```python
from build123d import *

# Parameters (mm, degrees)
CHANFREIN1_SIZE         = 3
CHANFREIN1_SIZE2        = 1.091910703
CONG_1_R                = 2
ENL_V_MAT_EXTRU_1_DEPTH = 3
ESQUISSE3_R             = 1.5
ENL_V_MAT_EXTRU_2_DEPTH = 3
ESQUISSE4_R             = 5
ESQUISSE4_R_2           = 1.5
ENL_V_MAT_EXTRU_3_DEPTH = 1


with BuildPart() as part:
    # Esquisse1 → Révolution1 (revolve)
    with BuildSketch(Plane.XY):
        Polygon((0, 23), (0, -20), (0, -22), (-1.5, -22), (-1.5, -20), (-15, -20), (-15, 5), (-5, 5), (-5, 10), (-1.5, 10), (-1.5, 23), align=None)
    revolve(axis=Axis((0, 23, 0), (0, -1, 0)))

    # Chanfrein1
    chanfrein1_edges = [part.edges().sort_by_distance(p)[0] for p in [
        (15, 5, 0),
    ]]
    chanfrein1_side = [part.faces().sort_by_distance(p)[0] for p in [
        (15, -7.5, 0),
    ]]
    chamfer(chanfrein1_edges, length=CHANFREIN1_SIZE, length2=CHANFREIN1_SIZE2, reference=chanfrein1_side[0])

    # Congé1
    cong_1_edges = [part.edges().sort_by_distance(p)[0] for p in [
        (15, -20, 0),
    ]]
    fillet(cong_1_edges, radius=CONG_1_R)

    # Esquisse2 → Enlèv. mat.-Extru.1 (cut)
    with BuildSketch(Plane(origin=(0, 5, 0), x_dir=(1, 0, 0), z_dir=(0, 1, 0))):
        with BuildLine():
            Line((-4, 9), (-4, 19))
            Line((-4, 19), (4, 19))
            Line((4, 19), (4, 9))
            ThreePointArc((4, 9), (0, 5), (-4, 9))
        make_face()
        with BuildLine():
            Line((9, 4), (19, 4))
            Line((19, 4), (19, -4))
            Line((19, -4), (9, -4))
            ThreePointArc((9, -4), (5, 0), (9, 4))
        make_face()
        with BuildLine():
            Line((4, -9), (4, -19))
            Line((4, -19), (-4, -19))
            Line((-4, -19), (-4, -9))
            ThreePointArc((-4, -9), (0, -5), (4, -9))
        make_face()
        with BuildLine():
            Line((-9, -4), (-19, -4))
            Line((-19, -4), (-19, 4))
            Line((-19, 4), (-9, 4))
            ThreePointArc((-9, 4), (-5, 0), (-9, -4))
        make_face()
    extrude(amount=-ENL_V_MAT_EXTRU_1_DEPTH, mode=Mode.SUBTRACT)

    # Esquisse3 → Enlèv. mat.-Extru.2 (cut)
    with BuildSketch(Plane.XZ.offset(20)):
        with Locations((0, 9)):
            Circle(ESQUISSE3_R)
        with Locations((0, -9)):
            Circle(ESQUISSE3_R)
        with Locations((9, 0)):
            Circle(ESQUISSE3_R)
        with Locations((-9, 0)):
            Circle(ESQUISSE3_R)
        with BuildLine():
            ThreePointArc((-15, 3), (-6.514718626, 6.514718626), (-3, 15))
            ThreePointArc((-3, 15), (-12.991965185, 12.991965185), (-15, 3))
        make_face()
        with BuildLine():
            ThreePointArc((3, 15), (6.514718626, 6.514718626), (15, 3))
            ThreePointArc((15, 3), (12.889510499, 12.889510499), (3, 15))
        make_face()
        with BuildLine():
            ThreePointArc((15, -3), (6.514718626, -6.514718626), (3, -15))
            ThreePointArc((3, -15), (12.652903184, -12.652903184), (15, -3))
        make_face()
        with BuildLine():
            ThreePointArc((-15, -3), (-6.514718626, -6.514718626), (-3, -15))
            ThreePointArc((-3, -15), (-12.726788918, -12.726788918), (-15, -3))
        make_face()
    extrude(amount=-ENL_V_MAT_EXTRU_2_DEPTH, mode=Mode.SUBTRACT)

    # Esquisse4 → Enlèv. mat.-Extru.3 (cut)
    with BuildSketch(Plane.XZ.offset(20)):
        with Locations(Location((0, 0, 0), (0, 0, 180))):
            Circle(ESQUISSE4_R)
        with Locations(Location((0, 0, 0), (0, 0, 180))):
            Circle(ESQUISSE4_R_2, mode=Mode.SUBTRACT)
    extrude(amount=-ENL_V_MAT_EXTRU_3_DEPTH, mode=Mode.SUBTRACT)


solid = part.part
```
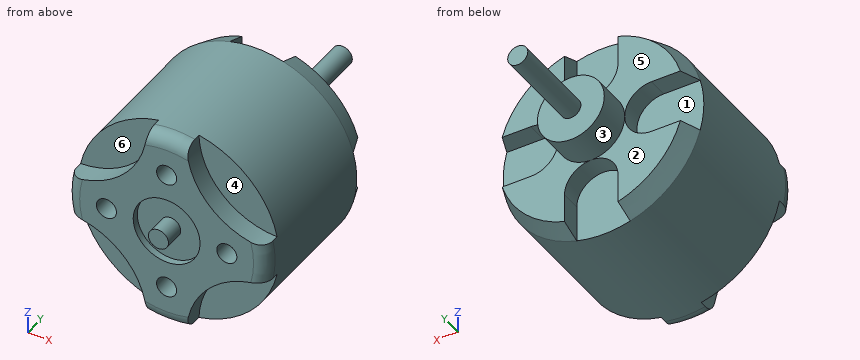
For this review, take the finished solid that the model builds, in its own axes (mm). Face numbers are marked on the shaded views. A direction names the side the tool comes from. Give positions to 0.01 mm unless a question says otherwise; leave off trailing zeros. Write each loop counter-clockwise with the first axis right and the second up, starting at its lowest first coordinate (ties: lowest second). Pieces come first, ordered by that corner, then holes.
Item 1: Wall thickness on probe 1 along Z at (x, y) = (10, -19); probe 2 along Y at (x, z) = (8, 5); probe 3 along Y at (x, z) = (-11, -4.5): over which ranges is each line inside the solid? List them lowest first.
Item 2: Take a section at B-B (y = 10.5). Give the boundary of the cut face in (x, z), and give its area (3 significant figures).
Item 3: Insertion check: P1, Ø2, axis at y = -8.5, z = -9, coming from the +X side; P2, Ø0.9, axis at x = -11, y = 3, coming from the -Z side; P3, Ø2.5, axis at y = 3.5, z = -11, coming from the -X side. Each pin has a flat end and moves straight along its axis. Give the tip position at first contact, or say it passes through.
Item 4: Take a section at A-A (y = -13.5). Give the boundary of the cut face in (x, z).
Item 5: Machinability: for the marked faces 4, 5 and 6, which of the approach directions +Z, -Z, +X, -X, +Y, -Y give a long, thin tool a straight path to every point of the face, cutting with its end or side? Answer none if there is none.
Item 6: The part is to be moulded in two halves that separate along Z. For the marked faces 1, 2 and 3, say which applies: +Z half, -Z half, draft (parallel to the pull), parting line (faces both ways), or undercut.
Established:
1. probe 1: z = -4.09 to -1.12, 1.12 to 4.09
1. probe 2: y = -20 to 5
1. probe 3: y = -17 to 5
2. outline: circle Ø3 at (0, 0)
2. area: 7.07 mm2
3. P1: stops at x = 12.69
3. P2: stops at z = -10.2
3. P3: stops at x = -10.83
4. outline: circle Ø30 at (0, 0)
5. face 4: +Z, +X, -Y
5. face 5: +Z, -X, +Y
5. face 6: +Z, -X, -Y
6. face 1: undercut
6. face 2: draft
6. face 3: parting line
